Read the model definition and answer for the solid it produces. Units are mm, in the model's axes. Face numbers are marked on the shaded views. A direction names the side the tool comes from. Give positions to 0.01 mm unless a question says otherwise; leave off trailing zeros. Loops run counter-clockwise (first coordinate to the right, second up) from the corner with the lowest first, then second, coordinate; pieces in that order, holes last. Notation, with made-up numbers: (76.5, 66) -> (113.5, 66) arc R30 cw to (113.5, 99) -> close; hole circle Ø1 at (7, 2). An arc over 180 degrees is marked (long way). Write each question's results on one line, items separated by ' | '. Start each with the question number.
Item 1: Find the intervals of material crossed by line 1 (X direction, y = 2.4, z = 0); line 2 (Y direction, x = 1, z = 0.25); line 3 (X direction, y = 2.4, z = 1.75), in increasing order.
Item 2: Which of the six approach directions +Z, -Z, +X, -X, +Y, -Y give full straight-line access (tool end or side, diameter ignored) to the marked faces 4 and 5?
Item 3: Section A-A on y = 1.95 is taken. Write down the section's boundary in (x, z), and give its area (3 significant figures).
Item 4: Determine the mould class of the marked faces 1, 2 and 3 for opening direction Z: +Z half, -Z half, draft (parallel to the pull), parting line (faces both ways), or undercut.
Item 5: Section B-B on z = 0.5 is taken. State how many separate pieces and enclosed holes the cut face has, and give its area (3 significant figures).
Item 6: Section C-C on y = 0.6 is taken. Write down the section's boundary in (x, z), and give its area (3 significant figures).
Item 7: Each of these flat-tipped pins is pushed along its axis until it touches: P1, Ø1.8, axis at x = 4.75, z = 0, coming from the -Y side; P2, Ø5.5, axis at x = 0, z = 0, coming from the +Y side. Where does it stop, or does it pass through?
```python
from build123d import *

# Parameters (mm, degrees)
CHAMFER2_SIZE     = 0.5
CIRPATTERN1_COUNT = 2
CHAMFER3_SIZE     = 0.7
FILLET2_R         = 0.2


with BuildPart() as part:
    # Sketch1 → Revolve1 (revolve)
    with BuildSketch(Plane.XY, mode=Mode.PRIVATE) as revolve1_sk:
        Polygon((0, 0), (-7.25, 0), (-7.25, 3.2), (-3.1, 3.2), (-3.1, 1), (0, 1), align=None)
    revolve(revolve1_sk.sketch.rotate(Axis((0, 0, 0), (0, 1, 0)), 270), axis=Axis((0, 0, 0), (0, 1, 0)))

    # Chamfer2
    chamfer2_edges = [part.edges().sort_by_distance(p)[0] for p in [
        (0, 3.2, 3.1),
    ]]
    chamfer(chamfer2_edges, length=CHAMFER2_SIZE)

    # Sketch4 → CSK for M2 Flat Head Machine Screw1 (revolve, cut)
    with BuildSketch(Plane(origin=(-4.75, 0, 0), x_dir=(0, 0, -1), z_dir=(1, 0, 0))):
        Polygon((0, 0), (0, 5.660946681), (1.1, 5), (1.1, 1.1), (2.2, 0), align=None)
    csk_for_m2_flat_head_machine_screw1 = revolve(axis=Axis((-4.75, -6.35, 0), (0, 1, 0)), mode=Mode.SUBTRACT)

    # CirPattern1: CSK for M2 Flat Head Machine Screw1 ×2 about axis
    cirpattern1_axis = Axis((0, 0, 0), (0, 1, 0))
    for i in range(1, CIRPATTERN1_COUNT):
        add(csk_for_m2_flat_head_machine_screw1.rotate(cirpattern1_axis, i * 360 / CIRPATTERN1_COUNT), mode=Mode.SUBTRACT)

    # Chamfer3
    chamfer3_edges = [part.edges().sort_by_distance(p)[0] for p in [
        (0, 3.2, 7.25),
    ]]
    chamfer(chamfer3_edges, length=CHAMFER3_SIZE)

    # Fillet2
    fillet2_edges = [part.edges().sort_by_distance(p)[0] for p in [
        (0, 1, 3.1),
    ]]
    fillet(fillet2_edges, radius=FILLET2_R)


solid = part.part
```
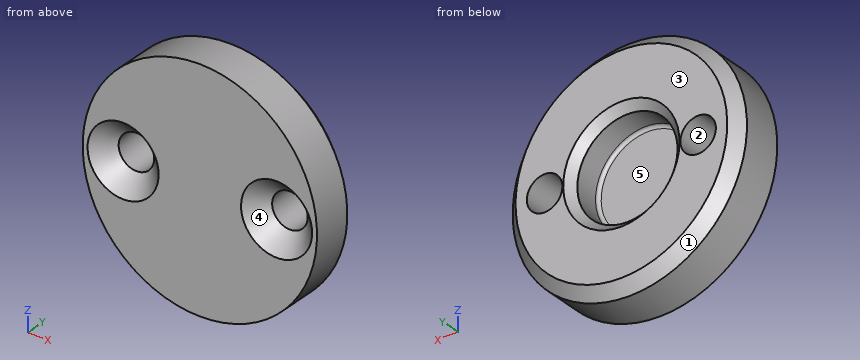
Findings:
1) line 1: -7.25 to -5.85, -3.65 to -3.1, 3.1 to 3.65, 5.85 to 7.25 | line 2: 0 to 1 | line 3: -7.04 to -2.56, 2.56 to 7.04
2) face 4: -Y | face 5: +Y
3) outline: circle Ø14.5 at (0, 0); hole circle Ø2.2 at (-4.75, 0); hole circle Ø6.2 at (0, 0); hole circle Ø2.2 at (4.75, 0) | area: 127 mm2
4) face 1: parting line | face 2: undercut | face 3: draft
5) separate pieces: 3 | enclosed holes: 0 | area: 17.0 mm2
6) outline: circle Ø14.5 at (0, 0); hole circle Ø3.2 at (-4.75, 0); hole circle Ø3.2 at (4.75, 0) | area: 149 mm2
7) P1: through | P2: y = 1
